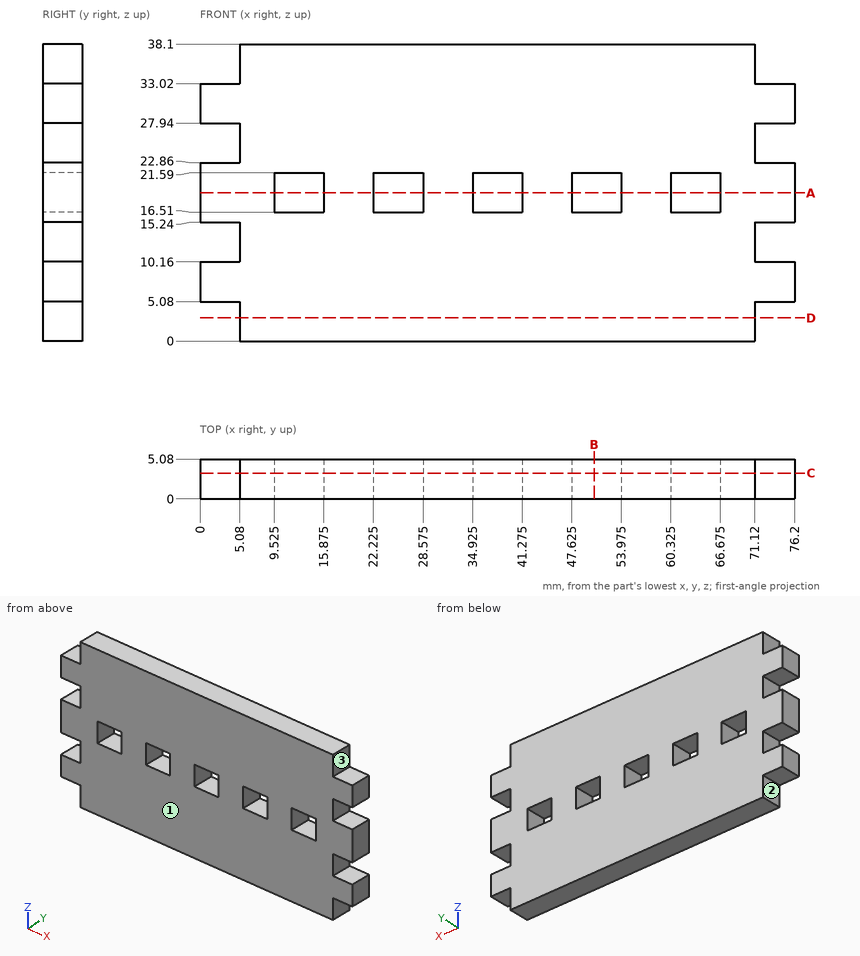
Geometry check sheet. Reference: drawing and pictorial views, mm from the part's lowest x, y, z. A direction names the side the tool comes from. Give positions to 0.01 mm unless a question says otherwise; leave off trailing zeros. Order: outer loops, then holes, each group sorted by start corner. A loop starts at its lowest first (then second) coordinate and runs counter-clockwise, first axis right, second up. Notation, with made-up numbers: (82.5, -9) - (112.5, -9) arc R11 cw to (112.5, 11) - close; hole circle Ø3 at (61.25, 45.25). An arc over 180 degrees is marked (long way). Answer as CSV lines item,"result".
1. Section check B-B (x = 50.5). Record the boundary of the cut face in (y, z), then the cut area to 3 significant figures.
Result sheet:
outline,"(0, 0) - (5.08, 0) - (5.08, 16.51) - (0, 16.51) - close; (0, 21.59) - (5.08, 21.59) - (5.08, 38.1) - (0, 38.1) - close"
area,"168 mm²"
2. Scan lines: probe 1 along X at (y, z) = (3.85, 18.5) (3 decimals); probe 2 along Z at (x, y) = (61, 1.25); probe 3 along X at (y, z) = (1.1, 25). Record each from-to range of solid material in increasing order. Write a range as from..to.
Result sheet:
probe 1,"0..9.525, 15.875..22.225, 28.575..34.925, 41.275..47.625, 53.975..60.325, 66.675..76.2"
probe 2,"0..16.51, 21.59..38.1"
probe 3,"5.08..71.12"
3. Tool access check on the marked faces 1, 2 and 3. Record the directions out of +Z, -Z, +X, -X, +Y, -Y that give a thin tool (end or side, any length) a straight path to the whole face; none if there is none.
Result sheet:
face 1,"+Z, -Z, +X, -X, -Y"
face 2,"-Z, -X, +Y, -Y"
face 3,"+Z, +X, +Y, -Y"
4. Section check A-A (z = 19). Record the boundary of the cut face in (x, y) (3 decimals), then the cut area to 3 significant figures.
Result sheet:
outline,"(0, 0) - (9.525, 0) - (9.525, 5.08) - (0, 5.08) - close; (15.875, 0) - (22.225, 0) - (22.225, 5.08) - (15.875, 5.08) - close; (28.575, 0) - (34.925, 0) - (34.925, 5.08) - (28.575, 5.08) - close; (41.275, 0) - (47.625, 0) - (47.625, 5.08) - (41.275, 5.08) - close; (53.975, 0) - (60.325, 0) - (60.325, 5.08) - (53.975, 5.08) - close; (66.675, 0) - (76.2, 0) - (76.2, 5.08) - (66.675, 5.08) - close"
area,"226 mm²"
5. Section check D-D (z = 3). Record the boundary of the cut face in (x, y).
Result sheet:
outline,"(5.08, 0) - (71.12, 0) - (71.12, 5.08) - (5.08, 5.08) - close"
6. Section check C-C (y = 3.3). State how many separate pieces and enclosed holes the cut face has, then the cut area to 3 significant figures.
Result sheet:
separate pieces,"1"
enclosed holes,"5"
area,"2,540 mm²"
7. Go/stop test with flat-tipped pins: P1, Ø12, axis at x = 30, z = 8, coming from the -Y side; P2, Ø2.5, axis at x = 3, y = 1.5, coming from the +Z side; P3, Ø1.5, axis at y = 2, z = 3.5, coming from the +X side. Record where each tip stops, or that it passes through.
Result sheet:
P1,"y = 0"
P2,"z = 33.02"
P3,"x = 71.12"
